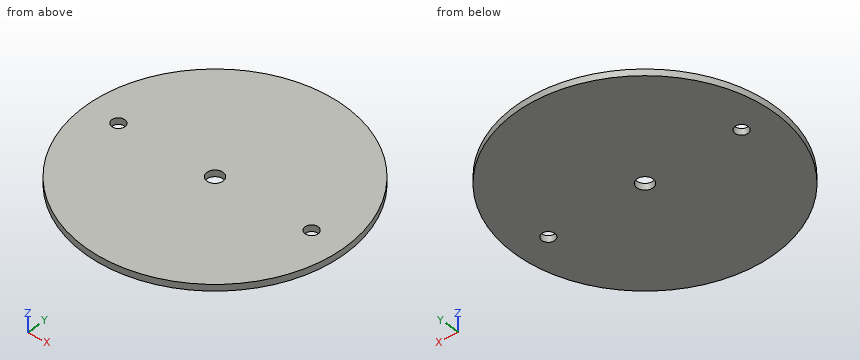
```python
from build123d import *

# Parameters (mm, degrees)
SKETCH1_R                          = 63.5
BOSS_EXTRUDE1_DEPTH                = 1.5875
F_1_4_0_25_DIAMETER_HOLE1_D        = 6.35
F_5_16_0_3125_DIAMETER_HOLE1_D     = 7.9375
F_5_16_0_3125_DIAMETER_HOLE1_DEPTH = 3.302


with BuildPart() as part:
    # Sketch1 → Boss-Extrude1 (new body, symmetric)
    with BuildSketch(Plane.XY):
        Circle(SKETCH1_R)
    extrude(amount=BOSS_EXTRUDE1_DEPTH, both=True)

    # 1/4 (0.25) Diameter Hole1 (through all)
    with Locations(Plane.XY.offset(1.5875)):
        with Locations((-47.625, 0), (47.625, 0)):
            Hole(F_1_4_0_25_DIAMETER_HOLE1_D / 2)

    # 5/16 (0.3125) Diameter Hole1
    with Locations(Plane.XY.offset(1.5875)):
        with Locations((0, 0)):
            Hole(F_5_16_0_3125_DIAMETER_HOLE1_D / 2, depth=F_5_16_0_3125_DIAMETER_HOLE1_DEPTH)


solid = part.part
```
CAD build for the part. Positions are in the model's coordinates, mm. Round coordinates to 2 decimals unless told otherwise and drop trailing zeros. Order: outer loops, then holes, each group sorted by start corner. A loop starts at its lowest first (then second) coordinate and runs counter-clockwise, first axis right, second up. Notation, with made-up numbers: (-19.5, 15) - (30.5, 15) arc R34 cw to (30.5, 50) - close; hole circle Ø9 at (52.5, 72.5). An arc over 180 degrees is marked (long way). Answer as CSV lines item,"result". Start each with the question number.
1. Saw through at D-D, the plane x = 39.5. Write the cut outline in (y, z).
2. Saw through at A-A, the plane y = 0. Write the cut outline in (x, z), and give its area (3 significant figures).
3. Saw through at C-C, the plane z = 0.55. Count the separate pieces of the cut face and the enclosed holes in it, and give its area (3 significant figures).
4. Saw through at B-B, the plane x = 0. Write the cut outline in (y, z).
5. Pin check, flat tip, straight feed: pin 1 (10.5 mm diameter, centred on x = 0, y = 0, fed in from +Z). Stop position of the tip, or through.
6. Drill centre lines: L1, parallel to Y at x = -48.5, z = 0.25; L2, parallel to Y at x = -5.5, z = -1.15; L3, parallel to X at y = 29, z = 0. Where is each one in solid material? Low to high. Write a range as [from, to].
Model answer:
1,outline,"(-49.72, -1.59) - (49.72, -1.59) - (49.72, 1.59) - (-49.72, 1.59) - close"
2,outline,"(-63.5, -1.59) - (-50.8, -1.59) - (-50.8, 1.59) - (-63.5, 1.59) - close; (-44.45, -1.59) - (-3.97, -1.59) - (-3.97, 1.59) - (-44.45, 1.59) - close; (3.97, -1.59) - (44.45, -1.59) - (44.45, 1.59) - (3.97, 1.59) - close; (50.8, -1.59) - (63.5, -1.59) - (63.5, 1.59) - (50.8, 1.59) - close"
2,area,"338 mm²"
3,separate pieces,"1"
3,enclosed holes,"3"
3,area,"12,600 mm²"
4,outline,"(-63.5, -1.59) - (-3.97, -1.59) - (-3.97, 1.59) - (-63.5, 1.59) - close; (3.97, -1.59) - (63.5, -1.59) - (63.5, 1.59) - (3.97, 1.59) - close"
5,pin 1,"stops at z = 1.59"
6,L1,"y = [-40.99, -3.05], [3.05, 40.99]"
6,L2,"y = [-63.26, 63.26]"
6,L3,"x = [-56.49, 56.49]"
